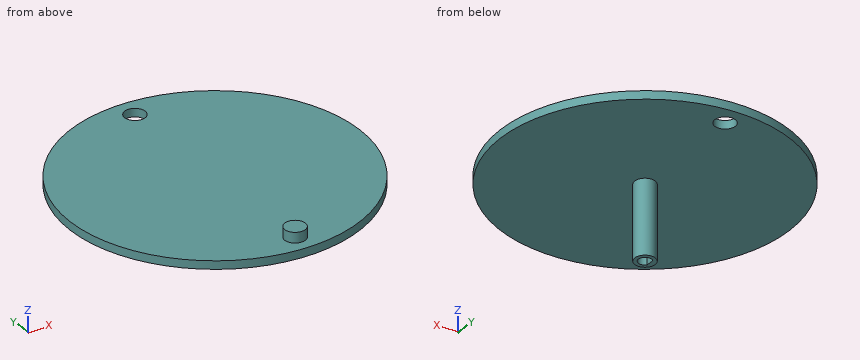
```python
from build123d import *

# Parameters (mm, degrees)
SKETCH1_R           = 88.9
SKETCH1_R_2         = 6
SKETCH1_R_3         = 6.35
BOSS_EXTRUDE1_DEPTH = 5.08
SKETCH2_R           = 6.35
BOSS_EXTRUDE2_DEPTH = 11.43
SKETCH3_R           = 6.35
BOSS_EXTRUDE3_DEPTH = 50.8
CUT_EXTRUDE1_DEPTH  = 18


with BuildPart() as part:
    # Sketch1 → Boss-Extrude1 (new body)
    with BuildSketch(Plane.XY):
        Circle(SKETCH1_R)
        Circle(SKETCH1_R_2, mode=Mode.SUBTRACT)
        with Locations((0, -76.2)):
            Circle(SKETCH1_R_3, mode=Mode.SUBTRACT)
        with Locations((0, 76.2)):
            Circle(SKETCH1_R_3, mode=Mode.SUBTRACT)
    extrude(amount=BOSS_EXTRUDE1_DEPTH)

    # Sketch2 → Boss-Extrude2 (add)
    with BuildSketch(Plane.XY):
        with Locations((0, -76.2)):
            Circle(SKETCH2_R)
    extrude(amount=BOSS_EXTRUDE2_DEPTH)

    # Sketch3 → Boss-Extrude3 (add)
    with BuildSketch(Plane.XY.offset(5.08)):
        Circle(SKETCH3_R)
    extrude(amount=-BOSS_EXTRUDE3_DEPTH)

    # Sketch4 → Cut-Extrude1 (cut)
    with BuildSketch(Plane(origin=(0, 0, -45.72), x_dir=(-1, 0, 0), z_dir=(0, 0, -1))):
        with BuildLine():
            Line((3.05, 2.664582519), (3.05, -2.664582519))
            ThreePointArc((3.05, -2.664582519), (-4.05, 0), (3.05, 2.664582519))
        make_face()
    extrude(amount=-CUT_EXTRUDE1_DEPTH, mode=Mode.SUBTRACT)


solid = part.part
```
Design review of the part built by this model. Coordinates are the model's own, in mm. Coordinates: 2 decimals unless noted, no trailing zeros. Loops run counter-clockwise (first coordinate to the right, second up) from the corner with the lowest first, then second, coordinate; pieces in that order, holes last. Notation, with made-up numbers: (-39, 69) -> (-7, 69) arc R14 ccw to (-7, 79) -> close; hole circle Ø2 at (-2.75, 50). An arc over 180 degrees is marked (long way). Answer as a JSON object with one key per item and string values.
Q1. Take a section at C-C on z = -39. Give the boundary of the cut face in (x, y), plus the area to 3 significant figures.
Answer block:
{"outline": "circle Ø12.7 at (0, 0); hole (-3.05, -2.66) arc R4.05 ccw (long way) to (-3.05, 2.66) -> close", "area": "78.8 mm^2"}
Q2. To check wall thickness, follow L1, parallel to Y at x = 0, z = 1.55; L2, parallel to Z at x = -39.5, y = -78; L3, parallel to X at y = 76, z = 2. State the ranges of each line that lie inside material, in increasing order.
Answer block:
{"L1": "y = -88.9 to 69.85, 82.55 to 88.9", "L2": "z = 0 to 5.08", "L3": "x = -46.12 to -6.35, 6.35 to 46.12"}
Q3. Take a section at D-D on z = -12.5. Give the boundary of the cut face in (x, y).
Answer block:
{"outline": "circle Ø12.7 at (0, 0)"}
Q4. Take a section at A-A on x = 0. Give the boundary of the cut face in (y, z).
Answer block:
{"outline": "(-88.9, 0) -> (-6.35, 0) -> (-6.35, -45.72) -> (-4.05, -45.72) -> (-4.05, -27.72) -> (4.05, -27.72) -> (4.05, -45.72) -> (6.35, -45.72) -> (6.35, 0) -> (69.85, 0) -> (69.85, 5.08) -> (-69.85, 5.08) -> (-69.85, 11.43) -> (-82.55, 11.43) -> (-82.55, 5.08) -> (-88.9, 5.08) -> close; (82.55, 0) -> (88.9, 0) -> (88.9, 5.08) -> (82.55, 5.08) -> close"}
Q5. Clearance check with flat-ended pins moving along their axes: pin 1 Ø10 at (y, z) = (49, 1) entering from -X; pin 2 Ø3 at (x, y) = (11, -44.5) entering from -Z; pin 3 Ø3 at (y, z) = (-7, -37.5) entering from -X. State where each tip first meets the part, or that it passes through.
Answer block:
{"pin 1": "stops at x = -77.25", "pin 2": "stops at z = 0", "pin 3": "stops at x = -3.17"}
Q6. Take a section at B-B on y = 0. Give the boundary of the cut face in (x, z), plus the area to 3 significant figures.
Answer block:
{"outline": "(-88.9, 0) -> (-6.35, 0) -> (-6.35, -45.72) -> (-3.05, -45.72) -> (-3.05, -27.72) -> (4.05, -27.72) -> (4.05, -45.72) -> (6.35, -45.72) -> (6.35, 0) -> (88.9, 0) -> (88.9, 5.08) -> (-88.9, 5.08) -> close", "area": "1,360 mm^2"}
